Check sheet for the modelled part. Datum: model origin and axes. Units: mm. A direction names the side the tool comes from. Give positions to 0.01 mm unless a question says otherwise; leave off trailing zeros. Order: outer loops, then holes, each group sorted by start corner. A loop starts at its lowest first (then second) coordinate and runs counter-clockwise, first axis right, second up.
```python
from build123d import *

# Parameters (mm, degrees)
CORTAR_EXTRUIR4_DEPTH      = 1
CROQUIS7_R                 = 7.5
CORTAR_EXTRUIR5_DEPTH      = 9
CORTAR_EXTRUIR6_DEPTH      = 9
CORTAR_EXTRUIR8_DEPTH      = 5
CORTAR_EXTRUIR8_DEPTH_BACK = 28.93644573
CROQUIS10_R                = 3
CROQUIS11_R                = 1.5
CORTAR_EXTRUIR9_DEPTH      = 5.2


with BuildPart() as part:
    # Croquis1 → Revolución1 (revolve)
    with BuildSketch(Plane(origin=(0, 0, 0), x_dir=(0, 0, -1), z_dir=(1, 0, 0))):
        Polygon((0, 0), (9.25, 0), (9.25, 10.25), (-12.25, 10.25), (-12.25, 10.95), (-12.95, 10.95), (-12.95, 0), align=None)
    revolve(axis=Axis((0, 0, 0), (0, 0, 1)))

    # Croquis5 → Cortar-Extruir4 (cut)
    with BuildSketch(Plane.XY.offset(12.95)):
        with BuildLine():
            ThreePointArc((-1.4, 4.276680956), (0, 4.5), (1.4, 4.276680956))
            Line((1.4, 4.276680956), (4.4, 8.276680956))
            ThreePointArc((4.4, 8.276680956), (0, 8.95), (-4.4, 8.276680956))
            Line((-4.4, 8.276680956), (-1.4, 4.276680956))
        make_face()
        with BuildLine():
            Line((4.967815967, 7.948852255), (3.003714352, 3.350776043))
            ThreePointArc((3.003714352, 3.350776043), (3.897114317, 2.25), (4.403714352, 0.925904913))
            Line((4.403714352, 0.925904913), (9.367815967, 0.327828701))
            ThreePointArc((9.367815967, 0.327828701), (7.750927364, 4.475), (4.967815967, 7.948852255))
        make_face()
        with BuildLine():
            Line((9.367815967, -0.327828701), (4.403714352, -0.925904913))
            ThreePointArc((4.403714352, -0.925904913), (3.897114317, -2.25), (3.003714352, -3.350776043))
            Line((3.003714352, -3.350776043), (4.967815967, -7.948852255))
            ThreePointArc((4.967815967, -7.948852255), (7.750927364, -4.475), (9.367815967, -0.327828701))
        make_face()
        with BuildLine():
            Line((4.4, -8.276680956), (1.4, -4.276680956))
            ThreePointArc((1.4, -4.276680956), (0, -4.5), (-1.4, -4.276680956))
            Line((-1.4, -4.276680956), (-4.4, -8.276680956))
            ThreePointArc((-4.4, -8.276680956), (0, -8.95), (4.4, -8.276680956))
        make_face()
        with BuildLine():
            ThreePointArc((-3.003714352, -3.350776043), (-3.897114317, -2.25), (-4.403714352, -0.925904913))
            Line((-4.403714352, -0.925904913), (-9.367815967, -0.327828701))
            ThreePointArc((-9.367815967, -0.327828701), (-7.750927364, -4.475), (-4.967815967, -7.948852255))
            Line((-4.967815967, -7.948852255), (-3.003714352, -3.350776043))
        make_face()
        with BuildLine():
            ThreePointArc((-4.403714352, 0.925904913), (-3.897114317, 2.25), (-3.003714352, 3.350776043))
            Line((-3.003714352, 3.350776043), (-4.967815967, 7.948852255))
            ThreePointArc((-4.967815967, 7.948852255), (-7.750927364, 4.475), (-9.367815967, 0.327828701))
            Line((-9.367815967, 0.327828701), (-4.403714352, 0.925904913))
        make_face()
    extrude(amount=-CORTAR_EXTRUIR4_DEPTH, mode=Mode.SUBTRACT)

    # Croquis7 → Cortar-Extruir5 (cut)
    with BuildSketch(Plane(origin=(0, 0, -9.25), x_dir=(-1, 0, 0), z_dir=(0, 0, -1))):
        with Locations(Location((0, 0, 0), (0, 0, 90))):
            Circle(CROQUIS7_R)
    extrude(amount=-CORTAR_EXTRUIR5_DEPTH, mode=Mode.SUBTRACT)

    # Croquis8 → Cortar-Extruir6 (cut)
    with BuildSketch(Plane(origin=(0, 0, -0.25), x_dir=(-1, 0, 0), z_dir=(0, 0, -1))):
        with BuildLine():
            Line((-1.140175425, -1.05), (1.140175425, -1.05))
            ThreePointArc((1.140175425, -1.05), (0, 1.55), (-1.140175425, -1.05))
        make_face()
    extrude(amount=-CORTAR_EXTRUIR6_DEPTH, mode=Mode.SUBTRACT)

    # Croquis10 → Cortar-Extruir8 (cut, two sides: drawn at the far end of the back side and taken through both)
    with BuildSketch(Plane(origin=(0, -11.25, 0), x_dir=(1, 0, 0), z_dir=(0, 1, 0)).offset(-CORTAR_EXTRUIR8_DEPTH_BACK)):
        with Locations(Location((0, -5.75, 0), (0, 0, 90))):
            Circle(CROQUIS10_R)
    extrude(amount=CORTAR_EXTRUIR8_DEPTH + CORTAR_EXTRUIR8_DEPTH_BACK, mode=Mode.SUBTRACT)

    # Croquis11 → Cortar-Extruir9 (cut)
    with BuildSketch(Plane.XZ.offset(6.25)):
        with Locations(Location((0, 5.75, 0), (0, 0, 270))):
            Circle(CROQUIS11_R)
    extrude(amount=-CORTAR_EXTRUIR9_DEPTH, mode=Mode.SUBTRACT)

    # Croquis12 → Revolución3 (revolve)
    with BuildSketch(Plane(origin=(0, 0, 0), x_dir=(0, 0, -1), z_dir=(1, 0, 0)), mode=Mode.PRIVATE) as revoluci_n3_sk:
        Polygon((-12.25, 10.25), (-12.25, 14.25), (9.156518587, 14.25), (9.25, 10.25), align=None)
    revolve(revoluci_n3_sk.sketch.rotate(Axis((0, 0, 0), (0, 0, -1)), 90), axis=Axis((0, 0, 0), (0, 0, -1)))


solid = part.part
```
(1) Thickness scan on L1, parallel to Z at x = 0, y = -4; L2, parallel to Y at x = 0, z = 2.25; L3, parallel to Z at x = 7.25, y = -5. Record the ranges inside material, lowest first.
(2) Release check for a two-part mould opening along X. For faces 1 (the face through (6.66, -8.69, 12.6)), 2 (the face through (-3.91, 2.23, 12.46)) record: released by +X, released by -X, zero draft, split by the parting line, or undercut.
(3) Go/stop test with flat-tipped pins: P1, Ø3, axis at y = -9, z = 9.5, coming from the +X side; P2, Ø7.5, axis at x = -2, y = 1, coming from the -Z side; P3, Ø2.5, axis at x = 0.5, y = -6, coming from the +Z side. Record where each tip stops, or that it passes through.
(4) Sectioned sample at D-D (z = -5). Enter the section's corners in (x, y), plus the area to 3 significant figures.
(5) Sectioned sample at A-A (z = 5.75). Enter the section's corners in (x, y).
(6) Tool access check on faces 3 (the face through (0, -7, 11.95)), 4 (the face through (0.33, -7.493, -4.813)), 5 (the face through (1, -6.25, 4)). Record the directions out of +Z, -Z, +X, -X, +Y, -Y that give a thin tool (end or side, any length) a straight path to the whole face; none if there is none.
(7) Sectioned sample at C-C (z = 3.5). Enter the section's corners in (x, y).
Values follow:
1. L1: z = -0.25 to 4.25, 7.25 to 12.95
1. L2: y = -14.25 to -1.05, 1.55 to 14.25
1. L3: z = -9.25 to 11.95
2. face 1: split by the parting line
2. face 2: undercut
3. P1: stops at x = 12.12
3. P2: stops at z = -0.25
3. P3: stops at z = 11.95
4. outline: circle Ø28.5 at (0, 0); hole circle Ø15 at (0, 0)
4. area: 461 mm2
5. outline: circle Ø28.5 at (0, 0); hole (-3, -9.8) arc R10.25 ccw to (3, -9.8) - (3, -6.25) - (1.5, -6.25) - (1.5, -1.05) - (1.14, -1.05) arc R1.55 ccw (long way) to (-1.14, -1.05) - (-1.5, -1.05) - (-1.5, -6.25) - (-3, -6.25) - close
6. face 3: +Z
6. face 4: -Z
6. face 5: none
7. outline: circle Ø28.5 at (0, 0); hole (-1.98, -10.06) arc R10.25 ccw to (1.98, -10.06) - (1.98, -6.25) - (-1.98, -6.25) - close; hole (-1.14, -1.05) - (1.14, -1.05) arc R1.55 ccw (long way) to start
